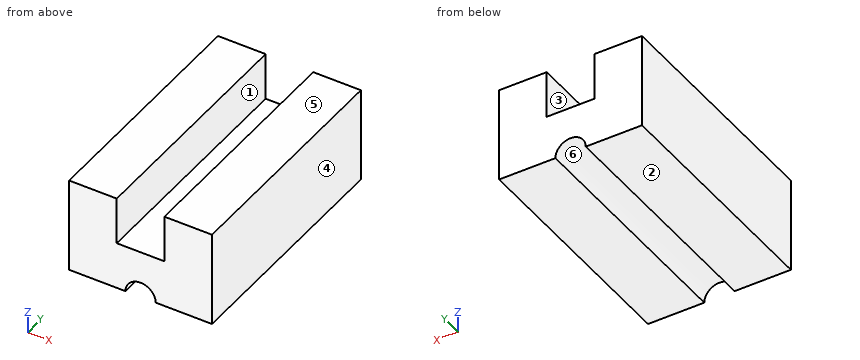
from build123d import *

# Parameters (mm, degrees)
F1_DEPTH = 12.7
F2_R     = 0.808299
F3_DEPTH = 25.4


with BuildPart() as f1:
    # F0 (on Front) → F1 (new body)
    with BuildSketch(Plane.XZ):
        Polygon((-1.27, 0.892354), (-3.81, 0.892354), (-3.81, -4.187646), (3.81, -4.187646), (3.81, 0.892354), (1.27, 0.892354), (1.27, -1.647646), (-1.27, -1.647646), align=None)
    extrude(amount=F1_DEPTH)

    # F2 (on face) → F3 (cut)
    with BuildSketch(Plane.XZ.offset(12.7)):
        with Locations((0, -4.187646)):
            Circle(F2_R)
    extrude(amount=-F3_DEPTH, mode=Mode.SUBTRACT)


solid = f1.part
Geometry check sheet. Reference: the model listing, model coordinates, mm. Face numbers are marked on the shaded views. A direction names the side the tool comes from. Coordinates: 2 decimals unless noted, no trailing zeros. Loops run counter-clockwise (first coordinate to the right, second up) from the corner with the lowest first, then second, coordinate; pieces in that order, holes last. Notation, with made-up numbers: (39.25, 61) - (49.25, 61) arc R12 ccw to (49.25, 79) - close; hole circle Ø1 at (64.5, 45). An arc over 180 degrees is marked (long way). Use one line per item in the form item = value. Start each with the question number.
Item 1: Mould release check, pull along X, two halves, no side actions. Record for the marked faces 3, 4, 5 and 6: +X half, -X half, draft (parallel to the pull), parting line (faces both ways), or undercut.
Item 2: Section check C-C, the plane x = 1. Enter the section's corners in (y, z).
Item 3: Section check A-A, the plane y = -7.75. Enter the section's corners in (x, z).
Item 4: Tool access check on the marked faces 1 and 2. Record the directions out of +Z, -Z, +X, -X, +Y, -Y that give a thin tool (end or side, any length) a straight path to the whole face; none if there is none.
Item 5: Section check B-B, the plane x = 0. Enter the section's corners in (y, z).
Item 6: Gauge pin test, flat ends, axial feed: pin 1 (3 mm diameter, centred on x = 1.5, z = -2.5, fed in from +Y); pin 2 (1.3 mm diameter, centred on x = 0.5, y = -8, fed in from +Z). Record the tip position at first contact, or that the pin passes through.
Item 7: Thickness scan on probe 1 along X at (y, z) = (-10.25, -0.45); probe 2 along X at (y, z) = (-6.75, -3.65); probe 3 along Z at (x, y) = (-1, -2.5). Record the ranges inside material, lowest first.
Computed:
q1.face_3 = undercut
q1.face_4 = +X half
q1.face_5 = draft
q1.face_6 = undercut
q2.outline = (-12.7, -4.19) - (0, -4.19) - (0, -1.65) - (-12.7, -1.65) - close
q3.outline = (-3.81, -4.19) - (-0.81, -4.19) arc R0.81 cw to (0.81, -4.19) - (3.81, -4.19) - (3.81, 0.89) - (1.27, 0.89) - (1.27, -1.65) - (-1.27, -1.65) - (-1.27, 0.89) - (-3.81, 0.89) - close
q4.face_1 = +Z, +Y, -Y
q4.face_2 = -Z, +X, -X, +Y, -Y
q5.outline = (-12.7, -3.38) - (0, -3.38) - (0, -1.65) - (-12.7, -1.65) - close
q6.pin_1 = 0
q6.pin_2 = -1.65
q7.probe_1 = -3.81 to -1.27, 1.27 to 3.81
q7.probe_2 = -3.81 to -0.6, 0.6 to 3.81
q7.probe_3 = -4.19 to -1.65
